from build123d import *


with BuildPart() as part:
    # Sketch2 → Revolve1 (revolve)
    with BuildSketch(Plane.XY, mode=Mode.PRIVATE) as revolve1_sk:
        Polygon((0, 0), (0, 9.220121932), (-11, 9.220121932), (-11, 7.720121932), (-10, 7.720121932), (-10, 6.220121932), (-12.006811328, 6.220121932), (-12.006811328, 4.370121932), align=None)
    revolve(revolve1_sk.sketch.rotate(Axis((0, 0, 0), (0, 1, 0)), 270), axis=Axis((0, 0, 0), (0, 1, 0)))

    # Sketch3 → Cut-Revolve1 (revolve, cut)
    with BuildSketch(Plane.XY, mode=Mode.PRIVATE) as cut_revolve1_sk:
        Polygon((0, 4.441105813), (0, 10.370121932), (-6, 10.370121932), (-6, 7.370121932), (-7.5, 7.370121932), (-7.5, 4.370121932), align=None)
    revolve(cut_revolve1_sk.sketch.rotate(Axis((0, 4.441105813, 0), (0, 1, 0)), 270), axis=Axis((0, 4.441105813, 0), (0, 1, 0)), mode=Mode.SUBTRACT)


solid = part.part
Input: part model. Units: mm. Frame: model coordinates. A direction names the side the tool comes from. Round coordinates to 2 decimals unless told otherwise and drop trailing zeros. Order: outer loops, then holes, each group sorted by start corner. A loop starts at its lowest first (then second) coordinate and runs counter-clockwise, first axis right, second up. Notation, with made-up numbers: (-13, 3) - (26, 3) arc R22 ccw to (26, 27) - close; hole circle Ø11 at (75.5, 56.5). An arc over 180 degrees is marked (long way). Use a Markdown table: item, result.
1. Material intervals for probe 1 along X at (y, z) = (8.45, 0); probe 2 along X at (y, z) = (6.75, 0.25); probe 3 along Z at (x, y) = (-1, 8.5), sorted ascending.
Evaluation:
| item | result |
|---|---|
| probe 1 | -11 to -6, 6 to 11 |
| probe 2 | -10 to -7.5, 7.5 to 10 |
| probe 3 | -10.95 to -5.92, 5.92 to 10.95 |
2. Access query for faces 1 (the face through (-1.802, 8.282, -5.723)), 2 (the face through (-6, 7.37, 2)), 3 (the face through (-8.115, 5.282, 8.85)). Directions: +Z, -Z, +X, -X, +Y, -Y. A direction counts if a zero-diameter tool reaches every point of the face in a straight line with its end or side. Return the directions, or none.
Evaluation:
| item | result |
|---|---|
| face 1 | +Y |
| face 2 | none |
| face 3 | +Y, -Y |
3. Mould query, pull axis Z, two halves, no side actions, for faces 4 (the face through (0.323, 4.438, -0.168)), 5 (the face through (10.74, 8.46, 2.38)), 6 (the face through (10, 7.72, -2)). Classes: +Z half, -Z half, draft (parallel to the pull), parting line (faces both ways), or undercut.
Evaluation:
| item | result |
|---|---|
| face 4 | undercut |
| face 5 | parting line |
| face 6 | draft |
4. First-contact query: pin 1 (1.5 mm diameter, centred on x = 9, z = 2, fed in from -Y); pin 2 (11 mm diameter, centred on x = 0, z = 0, fed in from +Y); pin 3 (5 mm diameter, centred on x = -1, z = -5, fed in from -Y). Flat tips, straight axial feed; report the tip coordinate or a pass-through.
Evaluation:
| item | result |
|---|---|
| pin 1 | y = 3.08 |
| pin 2 | y = 4.44 |
| pin 3 | y = 0.95 |
5. Section B-B on y = 0.5. Return the cut outline in (x, z), then the cut area to 3 significant figures.
Evaluation:
| item | result |
|---|---|
| outline | circle Ø2.75 at (0, 0) |
| area | 5.93 mm^2 |
6. Section A-A on y = 3.5. Return the cut outline in (x, z), then the cut area to 3 significant figures.
Evaluation:
| item | result |
|---|---|
| outline | circle Ø19.23 at (0, 0) |
| area | 291 mm^2 |
